Could you check a few things on this model? Use its own coordinates, in mm. A direction names the side the tool comes from. Coordinates: 2 decimals unless noted, no trailing zeros. Loops run counter-clockwise (first coordinate to the right, second up) from the corner with the lowest first, then second, coordinate; pieces in that order, holes last.
from build123d import *

# Parameters (mm, degrees)
F0_R     = 19.05
F1_DEPTH = 12.7
F2_R     = 8.6614
F3_DEPTH = 12.7
F4_SIZE  = 2.54
F7_R     = 3.175


with BuildPart() as f1:
    # F0 (on Top) → F1 (new body)
    with BuildSketch(Plane.XY):
        Circle(F0_R)
    extrude(amount=-F1_DEPTH)

    # F2 (on face) → F3 (join)
    with BuildSketch(Plane.XY):
        Circle(F2_R)
    extrude(amount=F3_DEPTH)

    # F4
    f4_edges = [f1.edges().sort_by_distance(p)[0] for p in [
        (-8.6614, 0, 12.7),
    ]]
    chamfer(f4_edges, length=F4_SIZE)

    # F5 (on Front) → F6 (revolve, cut)
    with BuildSketch(Plane.XZ):
        Polygon((19.05, -1.83179), (19.05, 0), (8.6614, 0), align=None)
    revolve(axis=Axis((0, 0, 4.455826), (0, 0, 1)), mode=Mode.SUBTRACT)

    # F7
    f7_edges = [f1.edges().sort_by_distance(p)[0] for p in [
        (-19.05, 0, -12.7),
    ]]
    fillet(f7_edges, radius=F7_R)


solid = f1.part
1) Imagine slicing it at D-D on z = -2.5. List the corners of the cut face in (x, y) for me, plus the area to 3 significant figures.
2) For faces 1 (the flat face through (0, 0, -12.7)), 2 (the cylindrical face through (3.997, -7.684, 5.009)), which set-ups out of +Z, -Z, +X, -X, +Y, -Y let a thin tool reach every point of the face, with its end or its side?
3) Imagine slicing it at A-A on x = 0. List the corners of the cut face in (y, z) for me (3 decimals).
4) If I drill on L1, parallel to X at y = -13, z = -5.5; L2, parallel to Z at x = -16, y = 2; L3, parallel to Z at x = -13.5, y = 11, over which ranges is the centre line in solid material (lowest first)?
5) Will these pins go through, and if not, where does the flat tip stop? pin 1 (3 mm diameter, centred on x = 9.5, z = 3.5, fed in from -Y); pin 2 (6 mm diameter, centred on x = 6.5, y = 11.5, fed in from +Z); pin 3 (3 mm diameter, centred on y = 1, z = 4, fed in from -X).
6) Imagine slicing it at C-C on z = 1.5. List the corners of the cut face in (x, y) for me, plus the area to 3 significant figures.
Solved:
1. outline: circle Ø38.1 at (0, 0)
1. area: 1,140 mm2
2. face 1: -Z, +X, -X, +Y, -Y
2. face 2: +Z
3. outline: (-19.05, -9.525) arc R3.175 ccw to (-15.875, -12.7) - (15.875, -12.7) arc R3.175 ccw to (19.05, -9.525) - (19.05, -1.832) - (8.661, 0) - (8.661, 10.16) - (6.121, 12.7) - (-6.121, 12.7) - (-8.661, 10.16) - (-8.661, 0) - (-19.05, -1.832) - close
4. L1: x = -13.92 to 13.92
4. L2: z = -12.69 to -1.32
4. L3: z = -12.3 to -1.54
5. pin 1: stops at y = -3.32
5. pin 2: stops at z = -0.27
5. pin 3: stops at x = -8.66
6. outline: circle Ø17.32 at (0, 0)
6. area: 236 mm2
